from build123d import *

# Parameters (mm, degrees)
SKETCH1_R           = 25
SKETCH1_R_2         = 4
SKETCH1_R_3         = 5
BOSS_EXTRUDE1_DEPTH = 10
SKETCH2_R           = 18
CUT_EXTRUDE1_DEPTH  = 4
SKETCH3_R           = 6
BOSS_EXTRUDE2_DEPTH = 1
SKETCH4_R           = 4
CUT_EXTRUDE2_DEPTH  = 13


with BuildPart() as part:
    # Sketch1 → Boss-Extrude1 (new body)
    with BuildSketch(Plane(origin=(0, 0, 0), x_dir=(1, 0, 0), z_dir=(0, 1, 0))):
        Circle(SKETCH1_R)
        Circle(SKETCH1_R_2, mode=Mode.SUBTRACT)
        with Locations((0, 12)):
            Circle(SKETCH1_R_3, mode=Mode.SUBTRACT)
        with Locations((12, 0)):
            Circle(SKETCH1_R_3, mode=Mode.SUBTRACT)
        with Locations((0, -12)):
            Circle(SKETCH1_R_3, mode=Mode.SUBTRACT)
        with Locations((-12, 0)):
            Circle(SKETCH1_R_3, mode=Mode.SUBTRACT)
    extrude(amount=BOSS_EXTRUDE1_DEPTH)

    # Sketch2 → Cut-Extrude1 (cut)
    with BuildSketch(Plane(origin=(0, 10, 0), x_dir=(1, 0, 0), z_dir=(0, 1, 0))):
        Circle(SKETCH2_R)
    extrude(amount=-CUT_EXTRUDE1_DEPTH, mode=Mode.SUBTRACT)

    # Sketch3 → Boss-Extrude2 (add)
    with BuildSketch(Plane.XZ):
        Circle(SKETCH3_R)
    extrude(amount=BOSS_EXTRUDE2_DEPTH)

    # Sketch4 → Cut-Extrude2 (cut)
    with BuildSketch(Plane(origin=(0, 0, 0), x_dir=(1, 0, 0), z_dir=(0, 1, 0))):
        Circle(SKETCH4_R)
    extrude(amount=-CUT_EXTRUDE2_DEPTH, mode=Mode.SUBTRACT)


solid = part.part
Here's how the part is built. I have some questions about the finished solid (model axes, mm). A direction names the side the tool comes from. Coordinates: 2 decimals unless noted, no trailing zeros. Order: outer loops, then holes, each group sorted by start corner. A loop starts at its lowest first (then second) coordinate and runs counter-clockwise, first axis right, second up. Notation, with made-up numbers: (23.25, 14.25) -> (72.25, 14.25) arc R22 ccw to (72.25, 29.25) -> close; hole circle Ø6 at (-4.5, 17). An arc over 180 degrees is marked (long way). Answer in a Markdown table with one row per item.
(1) Thinking about a two-plate mould opening in X: for faces 1 (the face through (5, 0, 5)), 2 (the face through (-4.3, 6, -0.3)), 3 (the face through (16.77, 2.96, -1.5)), 4 (the face through (-5.994, -0.493, 0.264)), which applies, +X half, -X half, draft (parallel to the pull), parting line (faces both ways), or undercut?
Answer key:
| item | result |
|---|---|
| face 1 | draft |
| face 2 | undercut |
| face 3 | undercut |
| face 4 | parting line |
(2) I want a section at C-C on z = 9. List the corners of the cut face in (x, y) for me, then the cut area to 3 significant figures.
Answer key:
| item | result |
|---|---|
| outline | (-23.32, 0) -> (-4, 0) -> (-4, 6) -> (-15.59, 6) -> (-15.59, 10) -> (-23.32, 10) -> close; (4, 0) -> (23.32, 0) -> (23.32, 10) -> (15.59, 10) -> (15.59, 6) -> (4, 6) -> close |
| area | 294 mm^2 |
(3) On a 3-axis mill with a long thin cutter (end or side, diameter ignored), from which of +Z, -Z, +X, -X, +Y, -Y can I reach the whole of each face in a straight line? I mean faces 5 (the face through (-0.651, 2.958, -16.957)), 6 (the face through (-2.343, 8.028, -17.847)). Say none if no direction works.
Answer key:
| item | result |
|---|---|
| face 5 | +Y, -Y |
| face 6 | +Y |
(4) I want a section at D-D on x = -12. List the corners of the cut face in (y, z) for me.
Answer key:
| item | result |
|---|---|
| outline | (0, -21.93) -> (10, -21.93) -> (10, -13.42) -> (6, -13.42) -> (6, -5) -> (0, -5) -> close; (0, 5) -> (6, 5) -> (6, 13.42) -> (10, 13.42) -> (10, 21.93) -> (0, 21.93) -> close |
(5) I want a section at A-A on x = 0. List the corners of the cut face in (y, z) for me.
Answer key:
| item | result |
|---|---|
| outline | (-1, -6) -> (0, -6) -> (0, -7) -> (6, -7) -> (6, -4) -> (-1, -4) -> close; (-1, 4) -> (6, 4) -> (6, 7) -> (0, 7) -> (0, 6) -> (-1, 6) -> close; (0, -25) -> (10, -25) -> (10, -18) -> (6, -18) -> (6, -17) -> (0, -17) -> close; (0, 17) -> (6, 17) -> (6, 18) -> (10, 18) -> (10, 25) -> (0, 25) -> close |
(6) I want a section at B-B on y = 1.75. List the corners of the cut face in (x, z) for me, then the cut area to 3 significant figures.
Answer key:
| item | result |
|---|---|
| outline | circle Ø50 at (0, 0); hole circle Ø10 at (-12, 0); hole circle Ø10 at (0, -12); hole circle Ø10 at (0, 12); hole circle Ø8 at (0, 0); hole circle Ø10 at (12, 0) |
| area | 1,600 mm^2 |
(7) Please list where these lines run through material, in increasing order: probe 1 along X at (y, z) = (2.25, 0); probe 2 along Z at (x, y) = (-4.5, 4.75).
Answer key:
| item | result |
|---|---|
| probe 1 | -25 to -17, -7 to -4, 4 to 7, 17 to 25 |
| probe 2 | -24.59 to -14.18, -9.82 to 9.82, 14.18 to 24.59 |
(8) Will these pins go through, and if not, where does the flat tip stop? pin 1 Ø4 at (x, y) = (-7.5, 3.5) entering from -Z; pin 2 Ø3 at (y, z) = (1.5, -11.5) entering from -X; pin 3 Ø2 at (x, z) = (-13, 6) entering from -Y.
Answer key:
| item | result |
|---|---|
| pin 1 | z = -24.39 |
| pin 2 | x = -22.91 |
| pin 3 | y = 0 |
